Part model, mm, in its own coordinate system. A direction names the side the tool comes from. Round coordinates to 2 decimals unless told otherwise and drop trailing zeros. Write each loop counter-clockwise with the first axis right and the second up, starting at its lowest first coordinate (ties: lowest second). Pieces come first, ordered by that corner, then holes.
1) Flat gauge pins, fed straight in: pin 1 (1.8 mm diameter, centred on x = 1, z = 25, fed in from -Y); pin 2 (1 mm diameter, centred on x = -7, y = 112.5, fed in from +Z); pin 3 (17.5 mm diameter, centred on x = -0.5, y = 163.5, fed in from -Z). Where does each tip first touch, or does it go through?
2) Saw through at C-C on x = 13. Write the cut outline in (y, z), and give its area (3 significant figures).
3) Which spindle directions (+Z, -Z, +X, -X, +Y, -Y) get a long thin tool onto all of the face, cutting with end or side? Do faces 4 (the flat face through (-7.016, 105.571, 20.846)), 5 (the cylindrical face through (-1.432, 154.094, 3.451)), 6 (the flat face through (8, 32, 8)). Say none if no direction does.
4) Pull direction X, two halves, no side cores. Call faces 1 (the flat face through (6.932, 105.571, 20.846)), 2 (the cylindrical face through (-0.65, 15.78, 21.07)), 3 (the flat face through (13, 178, 4)): +X half, -X half, draft (parallel to the pull), parting line (faces both ways), or undercut.
5) Saw through at A-A on x = 0. Write the cut outline in (y, z).
6) Drill centre lines: L1, parallel to Y at x = -2.5, z = 6; L2, parallel to Y at x = -10, z = 4; L3, parallel to Z at x = 0, y = 18. Where is each one in solid material? Low to high.
7) Saw through at B-B on x = -8. Write the cut outline in (y, z), and give its area (3 significant figures).
Autodesk Inventor part; units mm, degrees
ref_plane "Work Plane1" through (0, 28, 32) normal (0, -0.9898, 0.1423) x (1, 0, 0)
ref_plane "YZ Plane" through (0, 0, 0) normal (1, 0, 0) x (0, 1, 0)
ref_plane "XZ Plane" through (0, 0, 0) normal (0, 1, 0) x (-1, 0, 0)
sketch "Sketch1" plane through (0, 0, 0) normal (0, 0, 1) x (1, 0, 0)
  circle A0 centre (0, 165) radius 11
  line L0 (-11, 0) -> (-5, 0) construction
  line L1 (-5, 0) -> (-5, 24.6936) construction
  line L2 (-5, 24.6936) -> (-11, 24.6936) construction
  line L3 (-11, 24.6936) -> (-11, 0) construction
  line L4 (0, 0) -> (0, -33.6453) construction
  line L5 (11, 0) -> (5, 0) construction
  line L6 (5, 0) -> (5, 24.6936) construction
  line L7 (5, 24.6936) -> (11, 24.6936) construction
  line L8 (11, 24.6936) -> (11, 0) construction
  line L9 (16, 0) -> (-16, 0) construction
  line L10 (-16, 0) -> (-16, 181) construction
  line L11 (-16, 181) -> (16, 181) construction
  line L12 (16, 181) -> (16, 0) construction
  line L13 (-11, 168.4627) -> (-11, 161.5373) construction
  line L14 (-3.4627, 176) -> (3.4627, 176) construction
  point P0 (0, 0)
  point P1 (-11, 165)
  point P2 (0, 176)
  dimension "d0" = 22
  dimension "d1" = 165
  dimension "d2" = 6
  dimension "d3" = 10
  dimension "d4" = 5
  dimension "d8" = 5
  dimension "d9" = 5
  dimension "d10" = 32
sketch "Sketch2" plane through (0, 0, 0) normal (1, 0, 0) x (0, 1, 0)
  line L0 (0, 0) -> (181, 0)
  line L1 (181, 0) -> (181, 32) construction
  line L2 (181, 32) -> (0, 32) construction
  line L3 (0, 32) -> (0, 0)
  line L4 (0, 27) -> (25, 27)
  line L5 (25, 27) -> (25, 21)
  line L6 (25, 21) -> (0, 21)
  line L7 (0, 21) -> (0, 27)
  line L8 (25, 11) -> (0, 11)
  line L9 (0, 11) -> (0, 5)
  line L10 (0, 5) -> (25, 5)
  line L11 (25, 5) -> (25, 11)
  line L12 (0, 32) -> (28, 32)
  line L13 (176, 0) -> (154, 0)
  line L14 (176, 0) -> (154, 0) construction
  line L15 (154, 0) -> (154, 7) construction
  line L16 (154, 7) -> (176, 7) construction
  line L17 (176, 7) -> (176, 0) construction
  line L18 (181, 0) -> (181, 10)
  line L19 (181, 10) -> (28, 32)
  dimension "d7" = 32
  dimension "d11" = 6
  dimension "d12" = 10
  dimension "d13" = 5
  dimension "d14" = 25
  dimension "d15" = 7
  dimension "d16" = 3
  dimension "d17" = 3
extrude "Extrusion1" add sketch "Sketch2" along normal mid plane 32
chamfer "Chamfer1" distance 6 angle 45 6 edges at (-16, 104.5, 21) (-16, 14, 32) (16, 14, 32) (16, 104.5, 21) (-16, 181, 5) (16, 181, 5)
extrude "Extrusion2" cut sketch "Sketch1" along normal blind 7
sketch "Sketch3" plane through (-10, 181, 10) normal (0, 0.1423, 0.9898) x (1, 0, 0)
  line L0 (0, 0) -> (20, 0)
  line L1 (10, 0) -> (10, -154.5736)
  line L2 (0, -154.5736) -> (20, -154.5736)
  point P0 (10, -177.7341)
ref_plane "Work Plane1" through (0, 28, 32) normal (0, -0.9898, 0.1423) x (1, 0, 0)
sketch "Sketch4" plane through (0, 28, 32) normal (0, -0.9898, 0.1423) x (1, 0, 0)
  circle A0 centre (0, 3.4008) radius 5.2132
  point P0 (0, -35.6594)
extrude "Extrusion3" cut sketch "Sketch4" against normal through all both and the other way through all
sketch "Sketch5" plane through (-16, 0, 0) normal (0, -1, 0) x (1, 0, 0)
  circle A0 centre (8, 8) radius 3
  circle A1 centre (24, 8) radius 3
  circle A2 centre (16, 24) radius 3
  line L0 (32, 0) -> (0, 0)
  line L1 (24, 8) -> (8, 8) construction
  point P0 (16, 0)
  point P1 (16, 0)
  point P2 (16, 8)
  point P3 (16, 0)
  dimension "d27" = 6
  dimension "d28" = 16
  dimension "d29" = 8
  dimension "d30" = 16
extrude "Extrusion4" cut sketch "Sketch5" against normal blind 32
thread "Thread1"
thread "Thread2"
thread "Thread3"
equation "\"d4\" = 0.5 * d3"
equation "\"d18\" = d10"
equation "\"d30\" = d28"
equation "\"d31\" = d10"
properties part number "GB-stand"
Completed:
1. pin 1: stops at y = 32
1. pin 2: stops at z = 19.92
1. pin 3: stops at z = 7
2. outline: (0, 0) - (178, 0) - (178, 7.4) - (27.79, 29) - (0, 29) - close
2. area: 3,540 mm2
3. face 4: +Z, +X, -X, +Y
3. face 5: -Z
3. face 6: -Y
4. face 1: draft
4. face 2: undercut
4. face 3: +X half
5. outline: (0, 0) - (154, 0) - (154, 7) - (176, 7) - (176, 0) - (181, 0) - (181, 8.17) - (15.26, 32) - (0, 32) - (0, 27) - (32, 27) - (32, 21) - (0, 21) - close
6. L1: y = 0 to 154.29, 175.71 to 181
6. L2: y = 0 to 160.42, 169.58 to 181
6. L3: z = 0 to 21, 27 to 31.61
7. outline: (0, 0) - (157.45, 0) - (157.45, 7) - (172.55, 7) - (172.55, 0) - (181, 0) - (181, 10) - (28, 32) - (0, 32) - (0, 11) - (32, 11) - (32, 5) - (0, 5) - close
7. area: 3,810 mm2
